Design review of the part shown in the three views and the two pictorial views. Dimensions are in mm from the part's minimum x, y and z. A direction names the side the tool comes from. Give positions to 0.01 mm unless a question says otherwise; leave off trailing zeros. Loops run counter-clockwise (first coordinate to the right, second up) from the corner with the lowest first, then second, coordinate; pieces in that order, holes last. Notation, with made-up numbers: (15, 54.25) - (25, 54.25) arc R23 cw to (25, 69.25) - close; hole circle Ø11 at (64, 76). An arc over 180 degrees is marked (long way). Answer as a JSON object with one key per item and string values.
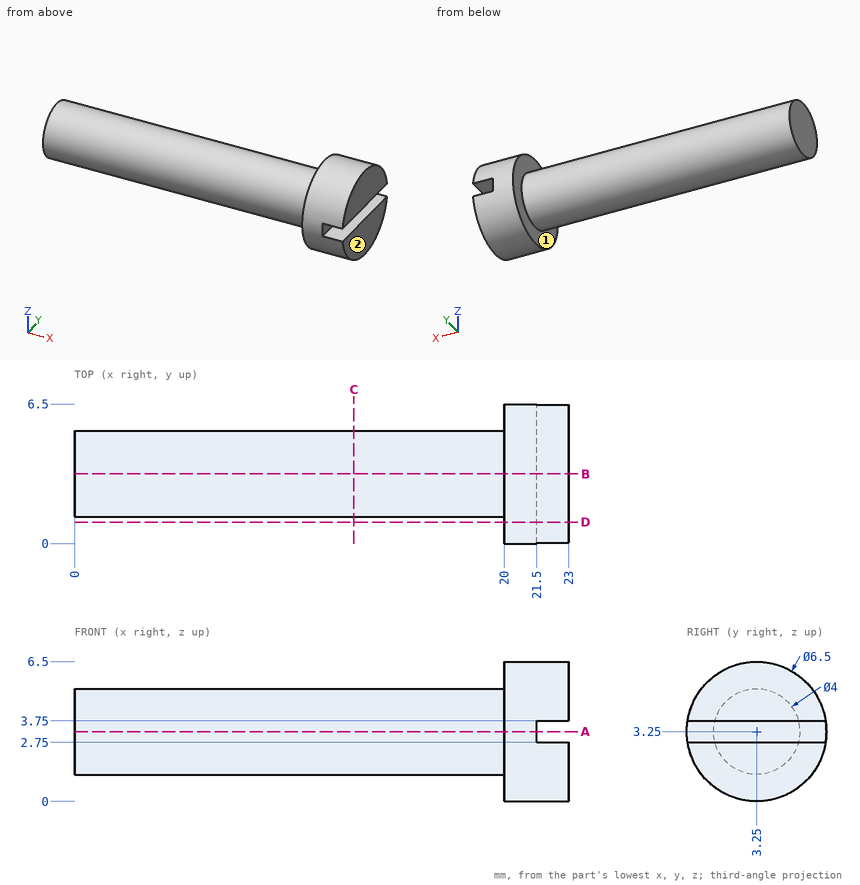
Q1. Clearance check with flat-ended pins moving along their axes: pin 1 Ø2 at (x, y) = (11, 4) entering from -Z; pin 2 Ø2 at (x, z) = (12, 4.5) entering from +Y; pin 3 Ø1.5 at (x, z) = (12, 5) entering from +Y. State where each tip first meets the part, or that it passes through.
Results:
{"pin 1": "stops at z = 1.25", "pin 2": "stops at y = 5.23", "pin 3": "stops at y = 4.98"}
Q2. Consider section C-C, the plane x = 13. State the section outline as (y, z) points.
Results:
{"outline": "circle Ø4 at (3.25, 3.25)"}
Q3. Consider section A-A, the plane z = 3.25. State the section outline as (x, y) points.
Results:
{"outline": "(0, 1.25) - (20, 1.25) - (20, 0) - (21.5, 0) - (21.5, 6.5) - (20, 6.5) - (20, 5.25) - (0, 5.25) - close"}
Q4. Consider section B-B, the plane y = 3.25. State the section outline as (x, z) points.
Results:
{"outline": "(0, 1.25) - (20, 1.25) - (20, 0) - (23, 0) - (23, 2.75) - (21.5, 2.75) - (21.5, 3.75) - (23, 3.75) - (23, 6.5) - (20, 6.5) - (20, 5.25) - (0, 5.25) - close"}
Q5. Consider section D-D, the plane y = 1. State the section outline as (x, z) points, plus the area to 3 significant figures.
Results:
{"outline": "(20, 0.9) - (23, 0.9) - (23, 2.75) - (21.5, 2.75) - (21.5, 3.75) - (23, 3.75) - (23, 5.6) - (20, 5.6) - close", "area": "12.6 mm^2"}
Q6. To check wall thickness, follow probe 1 along X at (y, z) = (4, 5.25); probe 2 along X at (y, z) = (2.5, 3.25); probe 3 along Z at (x, y) = (4.75, 1.5). State the ranges of each line that lie inside material, in increasing order. Write a range as [from, to].
Results:
{"probe 1": "x = [20, 23]", "probe 2": "x = [0, 21.5]", "probe 3": "z = [2.28, 4.22]"}
Q7. For the marked faces 1 and 2, list the 3-axis set-ups (+Z, -Z, +X, -X, +Y, -Y) from which the entire face can be reached by the end or side of a thin tool; tool diameter is ignored.
Results:
{"face 1": "-X", "face 2": "+Z, -Z, +X, +Y, -Y"}
